Check sheet for the modelled part. Datum: model origin and axes. Units: mm. Coordinates: 2 decimals unless noted, no trailing zeros. Write each loop counter-clockwise with the first axis right and the second up, starting at its lowest first coordinate (ties: lowest second). Pieces come first, ordered by that corner, then holes. Notation, with made-up numbers: (87.5, 4) - (145.5, 4) arc R20 cw to (145.5, 14) - close; hole circle Ø5 at (69.5, 49.5). An arc over 180 degrees is marked (long way). Use one line per item in the form item = value. Start each with the question number.
1. Cross-section at B-B on x = 15.24. Record the boundary of the cut face in (y, z) (3 decimals).
2. Cross-section at C-C on y = -2.5. Give the number of separate pieces and of enclosed holes in the cut face, then the cut area to 3 significant figures.
3. Scan lines: line 1 along Z through (x, y) = (0, -2.25); line 2 along Z through (x, y) = (-14, -2.75); line 3 along X through (y, z) = (-1.45, 5.5). Record each from-to range of solid material in increasing order.
4. Draft check along X on faces 1 (the face through (24.348, -1.565, 7.668)), 2 (the face through (11, 0, 0)), 3 (the face through (17.9, -1.6, 0.8)). Enter one of: +X half, -X half, draft (parallel to the pull), parting line (faces both ways), or undercut.
5. Go/stop test with a flat-tipped pin: pin 1 Ø1.5 at (x, y) = (-1, -1) entering from -Z. Record where the tip stops, or that it passes through.
6. Cross-section at D-D on x = 9.5. Record the boundary of the cut face in (y, z) (3 decimals).
7. Cross-section at A-A on z = -7. Record the boundary of the cut face in (x, y) (3 decimals).
```python
from build123d import *

# Parameters (mm, degrees)
F0_R     = 25.527
F0_R_2   = 2.778125
F1_DEPTH = 3.175


with BuildPart() as f1:
    # F0 (on Front) → F1 (new body)
    with BuildSketch(Plane.XZ):
        Circle(F0_R)
        with Locations((-7.62, -13.1982271537)):
            Circle(F0_R_2, mode=Mode.SUBTRACT)
        with Locations((-13.1982271537, -7.62)):
            Circle(F0_R_2, mode=Mode.SUBTRACT)
        with Locations((0, -15.24)):
            Circle(F0_R_2, mode=Mode.SUBTRACT)
        with Locations((7.62, -13.1982271537)):
            Circle(F0_R_2, mode=Mode.SUBTRACT)
        with Locations((13.1982271537, -7.62)):
            Circle(F0_R_2, mode=Mode.SUBTRACT)
        with Locations((-15.24, 0)):
            Circle(F0_R_2, mode=Mode.SUBTRACT)
        with Locations((-13.1982271537, 7.62)):
            Circle(F0_R_2, mode=Mode.SUBTRACT)
        with Locations((-7.62, 13.1982271537)):
            Circle(F0_R_2, mode=Mode.SUBTRACT)
        with BuildLine():
            ThreePointArc((8.89, 0), (-6.2861792847, -6.2861792847), (0, 8.89))
            ThreePointArc((0, 8.89), (6.2861792847, 6.2861792847), (8.89, 0))
        make_face(mode=Mode.SUBTRACT)
        with Locations((15.24, 0)):
            Circle(F0_R_2, mode=Mode.SUBTRACT)
        with Locations((13.1982271537, 7.62)):
            Circle(F0_R_2, mode=Mode.SUBTRACT)
        with BuildLine():
            ThreePointArc((0, 12.461875), (-1.9644310265, 17.2044310265), (2.778125, 15.24))
            ThreePointArc((2.778125, 15.24), (1.9644310265, 13.2755689735), (0, 12.461875))
        make_face(mode=Mode.SUBTRACT)
        with Locations((7.62, 13.1982271537)):
            Circle(F0_R_2, mode=Mode.SUBTRACT)
    extrude(amount=F1_DEPTH)


solid = f1.part
```
Final values:
q1.outline = (-3.175, -20.479) - (0, -20.479) - (0, -9.504) - (-3.175, -9.504) - close; (-3.175, -5.736) - (0, -5.736) - (0, -2.778) - (-3.175, -2.778) - close; (-3.175, 2.778) - (0, 2.778) - (0, 5.736) - (-3.175, 5.736) - close; (-3.175, 9.504) - (0, 9.504) - (0, 20.479) - (-3.175, 20.479) - close
q2.separate_pieces = 1
q2.enclosed_holes = 13
q2.area = 1,510 mm²
q3.line_1 = -25.53 to -18.02, -12.46 to -8.89, 8.89 to 12.46, 18.02 to 25.53
q3.line_2 = -21.35 to -10.28, -4.96 to -2.49, 2.49 to 4.96, 10.28 to 21.35
q3.line_3 = -24.93 to -14.99, -11.4 to -6.98, 6.98 to 11.4, 14.99 to 24.93
q4.face_1 = parting line
q4.face_2 = draft
q4.face_3 = undercut
q5.pin_1 = -25.53
q6.outline = (-3.175, -23.693) - (0, -23.693) - (0, -15.244) - (-3.175, -15.244) - close; (-3.175, -11.153) - (0, -11.153) - (0, 11.153) - (-3.175, 11.153) - close; (-3.175, 15.244) - (0, 15.244) - (0, 23.693) - (-3.175, 23.693) - close
q7.outline = (-24.548, -3.175) - (-15.906, -3.175) - (-15.906, 0) - (-24.548, 0) - close; (-10.49, -3.175) - (-5.48, -3.175) - (-5.48, 0) - (-10.49, 0) - close; (5.48, -3.175) - (10.49, -3.175) - (10.49, 0) - (5.48, 0) - close; (15.906, -3.175) - (24.548, -3.175) - (24.548, 0) - (15.906, 0) - close
